Verification items for the finished model (mm, model axes). Face numbers are marked on the shaded views. A direction names the side the tool comes from. Coordinates: 2 decimals unless noted, no trailing zeros. Order: outer loops, then holes, each group sorted by start corner. A loop starts at its lowest first (then second) coordinate and runs counter-clockwise, first axis right, second up. Notation, with made-up numbers: (-22.5, -19.5) - (11.5, -19.5) arc R27 ccw to (11.5, 10.5) - close; hole circle Ø7 at (78, 41). An arc over 180 degrees is marked (long way). Answer as CSV lines item,"result". Start each with the question number.
1. Go/stop test with flat-tipped pins: pin 1 (6 mm diameter, centred on y = 7, z = -12.5, fed in from -X); pin 2 (5 mm diameter, centred on x = 9.5, z = 3, fed in from +Y); pin 3 (1.5 mm diameter, centred on y = 5, z = 0.5, fed in from -X); pin 4 (5 mm diameter, centred on x = 3.5, y = 2, fed in from -Z). Record where each tip stops, or that it passes through.
2. Section check A-A (z = 1.5). Record the cut outline in (x, y), and give its area (3 significant figures).
3. Section check C-C (x = 6.75). Record the cut outline in (y, z), and give its area (3 significant figures).
4. Section check D-D (z = -29.5). Record the cut outline in (x, y), and give its area (3 significant figures).
5. Set-up check for the marked faces 1 and 2: record each of +Z, -Z, +X, -X, +Y, -Y from which the full face is reachable in a straight line by a thin tool's end or side.
6. Mould release check, pull along Y, two halves, no side actions. Record for the marked faces 3, 4 and 5: pulls with the +Y half, pulls with the -Y half, needs draft (parallel to the pull), parting line crosses it, or undercut.
7. Material ranges on L1, parallel to Y at x = 0, z = -4; L2, parallel to Z at x = 2, y = -10; L3, parallel to Y at x = 0, z = -47, recorded low to high. Write a range as [from, to].
8. Section check B-B (y = 9). Record the cut outline in (x, z), and give its area (3 significant figures).
from build123d import *

# Parameters (mm, degrees)
BASE_EXTRUSION_DEPTH    = 5
BOSS_EXTRU_1_DEPTH      = 0.5
ESQUISSE3_R             = 2.5
BOSS_EXTRU_2_DEPTH      = 5
BOSS_EXTRU_3_DEPTH      = 0.5
ESQUISSE5_R             = 6
BOSS_EXTRU_4_DEPTH      = 28
ESQUISSE6_R             = 3.5
BOSS_EXTRU_5_DEPTH      = 16
ESQUISSE7_R             = 3
BOSS_EXTRU_6_DEPTH      = 23
CHANFREIN1_SIZE         = 1
ESQUISSE8_R             = 4.25
ENL_V_MAT_EXTRU_1_DEPTH = 28
ENL_V_MAT_EXTRU_4_DEPTH = 4.25
CHANFREIN2_SIZE         = 0.5


with BuildPart() as part:
    # Esquisse1 → Base-Extrusion (new body)
    with BuildSketch(Plane.XY):
        with BuildLine():
            Line((2, 11.832159566), (7.5, 0))
            Line((7.5, 0), (12, 0))
            ThreePointArc((12, 0), (0, -12), (-12, 0))
            Line((-12, 0), (-7.5, 0))
            Line((-7.5, 0), (-2, 11.832159566))
            ThreePointArc((-2, 11.832159566), (0, 12), (2, 11.832159566))
        make_face()
    extrude(amount=BASE_EXTRUSION_DEPTH)

    # Esquisse2 → Boss.-Extru.1 (add)
    with BuildSketch(Plane.XY.offset(5)):
        with BuildLine():
            Line((2, 11.832159566), (4.148812154, 7.209416242))
            ThreePointArc((4.148812154, 7.209416242), (0, 5), (-4.148812154, 7.209416242))
            Line((-4.148812154, 7.209416242), (-2, 11.832159566))
            ThreePointArc((-2, 11.832159566), (0, 12), (2, 11.832159566))
        make_face()
    extrude(amount=BOSS_EXTRU_1_DEPTH)

    # Esquisse3 → Boss.-Extru.2 (add)
    with BuildSketch(Plane.XY.offset(5.5)):
        with Locations((0, 9)):
            Circle(ESQUISSE3_R)
    extrude(amount=BOSS_EXTRU_2_DEPTH)

    # Esquisse4 → Boss.-Extru.3 (add)
    with BuildSketch(Plane(origin=(0, 0, 0), x_dir=(-1, 0, 0), z_dir=(0, 0, -1))):
        with BuildLine():
            Line((-8, 0), (-7.5, 0))
            Line((-7.5, 0), (-4.391777187, 6.686725143))
            ThreePointArc((-4.391777187, 6.686725143), (0, 8), (4.391777187, 6.686725143))
            Line((4.391777187, 6.686725143), (7.5, 0))
            Line((7.5, 0), (8, 0))
            ThreePointArc((8, 0), (0, -8), (-8, 0))
        make_face()
    extrude(amount=BOSS_EXTRU_3_DEPTH)

    # Esquisse5 → Boss.-Extru.4 (add)
    with BuildSketch(Plane(origin=(0, 0, -0.5), x_dir=(-1, 0, 0), z_dir=(0, 0, -1))):
        Circle(ESQUISSE5_R)
    extrude(amount=BOSS_EXTRU_4_DEPTH)

    # Esquisse6 → Boss.-Extru.5 (add)
    with BuildSketch(Plane(origin=(0, 0, -28.5), x_dir=(-1, 0, 0), z_dir=(0, 0, -1))):
        Circle(ESQUISSE6_R)
    extrude(amount=BOSS_EXTRU_5_DEPTH)

    # Esquisse7 → Boss.-Extru.6 (add)
    with BuildSketch(Plane(origin=(0, 0, -44.5), x_dir=(-1, 0, 0), z_dir=(0, 0, -1))):
        Circle(ESQUISSE7_R)
    extrude(amount=BOSS_EXTRU_6_DEPTH)

    # Chanfrein1
    chanfrein1_edges = [part.edges().sort_by_distance(p)[0] for p in [
        (3, 0, -67.5),
    ]]
    chamfer(chanfrein1_edges, length=CHANFREIN1_SIZE)

    # Esquisse8 → Enlèv. mat.-Extru.1 (cut)
    with BuildSketch(Plane.XY.offset(5.5)):
        Circle(ESQUISSE8_R)
    extrude(amount=-ENL_V_MAT_EXTRU_1_DEPTH, mode=Mode.SUBTRACT)

    # Esquisse12 → Enlèv. mat.-Extru.4 (cut)
    with BuildSketch(Plane(origin=(4.242640687, 4.242640687, -14.5), x_dir=(-0.7071067811865462, 0.7071067811865489, 0), z_dir=(0.7071067811865489, 0.7071067811865462, 0))):
        with BuildLine():
            Line((-3.25, 6), (3.25, 6))
            ThreePointArc((3.25, 6), (3.957106781, 5.707106781), (4.25, 5))
            Line((4.25, 5), (4.25, -6))
            ThreePointArc((4.25, -6), (3.957106781, -6.707106781), (3.25, -7))
            Line((3.25, -7), (-3.25, -7))
            ThreePointArc((-3.25, -7), (-3.957106781, -6.707106781), (-4.25, -6))
            Line((-4.25, -6), (-4.25, 5))
            ThreePointArc((-4.25, 5), (-3.957106781, 5.707106781), (-3.25, 6))
        make_face()
    extrude(amount=-ENL_V_MAT_EXTRU_4_DEPTH, mode=Mode.SUBTRACT)

    # Chanfrein2
    chanfrein2_edges = [part.edges().sort_by_distance(p)[0] for p in [
        (-2.5, 9, 10.5),
    ]]
    chamfer(chanfrein2_edges, length=CHANFREIN2_SIZE)


solid = part.part
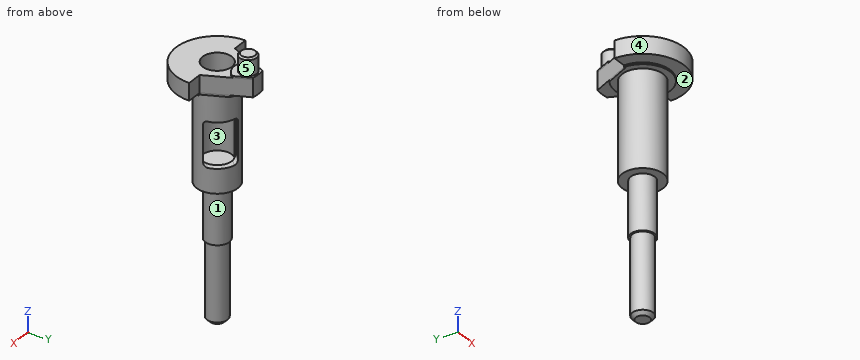
Evaluation:
1,pin 1,"stops at x = -4.47"
1,pin 2,"stops at y = 1.08"
1,pin 3,"stops at x = -5.52"
1,pin 4,"stops at z = -67.5"
2,outline,"(-12, 0) arc R12 ccw to (12, 0) - (7.5, 0) - (2, 11.83) arc R12 ccw to (-2, 11.83) - (-7.5, 0) - close; hole circle Ø8.5 at (0, 0)"
2,area,"282 mm²"
3,outline,"(-9.92, 0) - (-4.29, 0) - (-4.29, -0.5) - (1.61, -0.5) - (1.61, 5) - (-9.92, 5) - close"
3,area,"60.6 mm²"
4,outline,"circle Ø7 at (0, 0)"
4,area,"38.5 mm²"
5,face 1,"-Z"
5,face 2,"-Z, -Y"
6,face 3,"undercut"
6,face 4,"pulls with the -Y half"
6,face 5,"parting line crosses it"
7,L1,"y = [-6, -4.25], [4.25, 6]"
7,L2,"z = [0, 5]"
7,L3,"y = [-3, 3]"
8,outline,"(-3.32, 0) - (3.32, 0) - (3.32, 5.5) - (2.5, 5.5) - (2.5, 10) - (2, 10.5) - (-2, 10.5) - (-2.5, 10) - (-2.5, 5.5) - (-3.32, 5.5) - close"
8,area,"61.2 mm²"
